For this review, use the dimensioned drawing (mm, ordinates from the lowest corner) and the shaded views. A direction names the side the tool comes from. Coordinates: 2 decimals unless noted, no trailing zeros. Loops run counter-clockwise (first coordinate to the right, second up) from the corner with the lowest first, then second, coordinate; pieces in that order, holes last. Notation, with made-up numbers: M -19.5,8.5 L -12.5,8.5 A35 ccw -12.5,45.5 Z; hole C 36,-30.75 d6. An arc over 180 degrees is marked long. One line per item, written item: value.
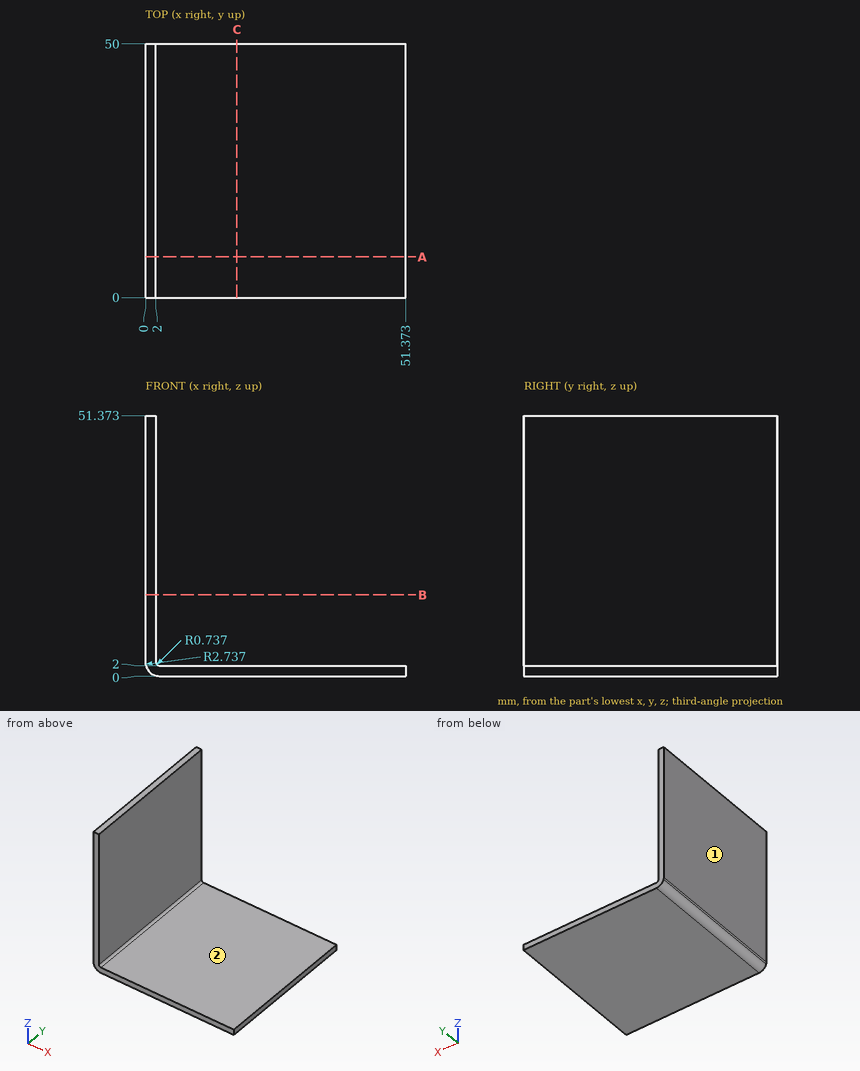
(1) We need section B-B on z = 16. State the section outline as (x, y) points.
Reply:
outline: M 0,0 L 2,0 L 2,50 L 0,50 Z
(2) We need section A-A on y = 8. State the section outline as (x, z) points.
Reply:
outline: M 0,2.74 A2.74 ccw 2.74,0 L 51.37,0 L 51.37,2 L 2.74,2 A0.74 cw 2,2.74 L 2,51.37 L 0,51.37 Z
(3) To check wall thickness, follow line 1 along X through (y, z) = (10.5, 29.5). State the ranges of the line that lie inside material, in increasing order. Write a range as [from, to].
Reply:
line 1: x = [0, 2]
(4) We need section C-C on x = 18. State the section outline as (y, z) points.
Reply:
outline: M 0,0 L 50,0 L 50,2 L 0,2 Z
(5) Tool access review of the marked faces 1 and 2: name each direction out of +Z, -Z, +X, -X, +Y, -Y from which nothing blocks a thin tool from reaching the whole face with its end or side.
Reply:
face 1: +Z, -Z, -X, +Y, -Y
face 2: +Z, +X, +Y, -Y
(6) Insertion check: pin 1 (10 mm diameter, centred on y = 42, z = 24.5, fed in from +X); pin 2 (3 mm diameter, centred on x = 33.5, y = 9.5, fed in from +Z). Each pin has a flat end and moves straight along its axis. Give the tip position at first contact, or say it passes through.
Reply:
pin 1: stops at x = 2
pin 2: stops at z = 2
